Read the model definition and answer for the solid it produces. Units are mm, in the model's axes. A direction names the side the tool comes from. Round coordinates to 2 decimals unless told otherwise and drop trailing zeros. Order: outer loops, then holes, each group sorted by start corner. A loop starts at its lowest first (then second) coordinate and runs counter-clockwise, first axis right, second up. Notation, with made-up numbers: (-13.5, -20.5) - (-7.5, -20.5) arc R33 ccw to (-7.5, 15.5) - close; hole circle Ø9 at (24, 57.5). An arc over 180 degrees is marked (long way). Answer as a JSON object with one key per item and string values. Group by question number.
Q1. Consider line 1 (Y direction, x = 7.5, z = 9); line 2 (Z direction, x = 2.5, y = 6). Determine where each line is inside the solid, lowest interval first.
Q2. A cutting plane is placed at A-A on x = 4.5. Determine the outline of the cut face in (y, z).
Q3. The mould has two halves that part along X. Classify faces 4 (the cylindrical face through (9.86, 0.582, -0.648)), 5 (the flat face through (20, 1, 9)), 6 (the flat face through (2.75, 1, 16)): pulls with the +X half, pulls with the -X half, needs draft (parallel to the pull), parting line crosses it, or undercut.
Q4. A cutting plane is placed at C-C on x = 2. Determine the outline of the cut face in (y, z).
Q5. A tool of negligible diameter and unlimited length cuts with its end or side. For faces 1 (the cylindrical face through (15.54, 0.61, 26.55)), 2 (the flat face through (10, 9, 0)), 3 (the flat face through (10, 15, -1)), from which of +Z, -Z, +X, -X, +Y, -Y can it reach the whole face along a straight path? Write none if from no direction.
Q6. Given pin 1 Ø4 at (x, y) = (7, 3.5) entering from +Z; pin 2 Ø10 at (x, z) = (17, 19) entering from +Y, each flat-ended and moving along its own axis, determine where each tip first touches the part or whether it passes through.
Q7. A cutting plane is placed at D-D on y = 2.5. Determine the outline of the cut face in (x, z).
Q8. A cutting plane is placed at B-B on z = 25.75. Determine the outline of the cut face in (x, y).
```python
from build123d import *

# Parameters (mm, degrees)
SKETCH_1_W                       = 20
SKETCH_1_H                       = 15
SM_BASE_FLANGE_1_DEPTH           = 1.2
SM_EDGE_FLANGE_1_STRIP_W         = 6.2732
SM_EDGE_FLANGE_1_STRIP_H         = 1.2
SM_EDGE_FLANGE_1_STRIP_CUT_DEPTH = 20
SM_EDGE_FLANGE_1_DEPTH           = 20
CUT_EXTRUDE_1_REACH              = 39.681


# Sheet-metal steps are written as plain solids
with BuildPart() as part:
    # Sketch 1 → Базовая кромка1 (new body)
    with BuildSketch(Plane.XY):
        with Locations((10, 7.5)):
            Rectangle(SKETCH_1_W, SKETCH_1_H)
    extrude(amount=-SM_BASE_FLANGE_1_DEPTH)

    # Ребро-кромка1 strip (across the edge) → Ребро-кромка1 strip cut (cut)
    with BuildSketch(Plane.YZ):
        with Locations((-1.2, -0.6)):
            Rectangle(SM_EDGE_FLANGE_1_STRIP_W, SM_EDGE_FLANGE_1_STRIP_H)
    extrude(amount=SM_EDGE_FLANGE_1_STRIP_CUT_DEPTH, mode=Mode.SUBTRACT)

    # Ребро-кромка1 section (across the edge) → Ребро-кромка1 (add)
    with BuildSketch(Plane.YZ):
        with BuildLine():
            Line((0, 0.7366), (0, 28.8))
            Line((0, 28.8), (1.2, 28.8))
            Line((1.2, 28.8), (1.2, 0.7366))
            ThreePointArc((1.2, 0.7366), (1.415745145, 0.215745145), (1.9366, 0))
            Line((1.9366, 0), (1.9366, -1.2))
            ThreePointArc((1.9366, -1.2), (0.567217008, -0.632782992), (0, 0.7366))
        make_face()
    extrude(amount=SM_EDGE_FLANGE_1_DEPTH)

    # Эскиз9 → Вырез-Вытянуть1 (cut, up to next)
    with BuildSketch(Plane(origin=(0, 1.2, 0), x_dir=(1, 0, 0), z_dir=(0, 1, 0)), mode=Mode.PRIVATE) as cut_extrude_1_sk1:
        with BuildLine():
            Line((6.25, -6.8), (6.25, -24.8))
            ThreePointArc((6.25, -24.8), (4.5, -26.55), (2.75, -24.8))
            Line((2.75, -24.8), (2.75, -6.8))
            ThreePointArc((2.75, -6.8), (4.5, -5.05), (6.25, -6.8))
        make_face()
    cut_extrude_1_tool1 = extrude(cut_extrude_1_sk1.sketch, amount=-CUT_EXTRUDE_1_REACH, mode=Mode.PRIVATE) & part.part
    # Эскиз9 → Вырез-Вытянуть1 (cut, up to next)
    with BuildSketch(Plane(origin=(0, 1.2, 0), x_dir=(1, 0, 0), z_dir=(0, 1, 0)), mode=Mode.PRIVATE) as cut_extrude_1_sk2:
        with BuildLine():
            Line((17.25, -6.8), (17.25, -24.8))
            ThreePointArc((17.25, -24.8), (15.5, -26.55), (13.75, -24.8))
            Line((13.75, -24.8), (13.75, -6.8))
            ThreePointArc((13.75, -6.8), (15.5, -5.05), (17.25, -6.8))
        make_face()
    cut_extrude_1_tool2 = extrude(cut_extrude_1_sk2.sketch, amount=-CUT_EXTRUDE_1_REACH, mode=Mode.PRIVATE) & part.part
    add(cut_extrude_1_tool1.solids().sort_by_distance((4.5, 1.2, 15.8))[0], mode=Mode.SUBTRACT)
    add(cut_extrude_1_tool2.solids().sort_by_distance((15.5, 1.2, 15.8))[0], mode=Mode.SUBTRACT)


solid = part.part
```
Result set:
{
 "1": {"line 1": "y = 0 to 1.2", "line 2": "z = -1.2 to 0"},
 "2": {"outline": "(0, 0.74) arc R1.94 ccw to (1.94, -1.2) - (15, -1.2) - (15, 0) - (1.94, 0) arc R0.74 cw to (1.2, 0.74) - (1.2, 5.05) - (0, 5.05) - close; (0, 26.55) - (1.2, 26.55) - (1.2, 28.8) - (0, 28.8) - close"},
 "3": {"face 4": "needs draft", "face 5": "pulls with the +X half", "face 6": "undercut"},
 "4": {"outline": "(0, 0.74) arc R1.94 ccw to (1.94, -1.2) - (15, -1.2) - (15, 0) - (1.94, 0) arc R0.74 cw to (1.2, 0.74) - (1.2, 28.8) - (0, 28.8) - close"},
 "5": {"face 1": "+Y, -Y", "face 2": "+Z, +X, -X, +Y", "face 3": "+Z, -Z, +X, -X, +Y"},
 "6": {"pin 1": "stops at z = 0.14", "pin 2": "stops at y = 1.2"},
 "7": {"outline": "(0, -1.2) - (20, -1.2) - (20, 0) - (0, 0) - close"},
 "8": {"outline": "(0, 0) - (3.03, 0) - (3.03, 1.2) - (0, 1.2) - close; (5.97, 0) - (14.03, 0) - (14.03, 1.2) - (5.97, 1.2) - close; (16.97, 0) - (20, 0) - (20, 1.2) - (16.97, 1.2) - close"}
}
